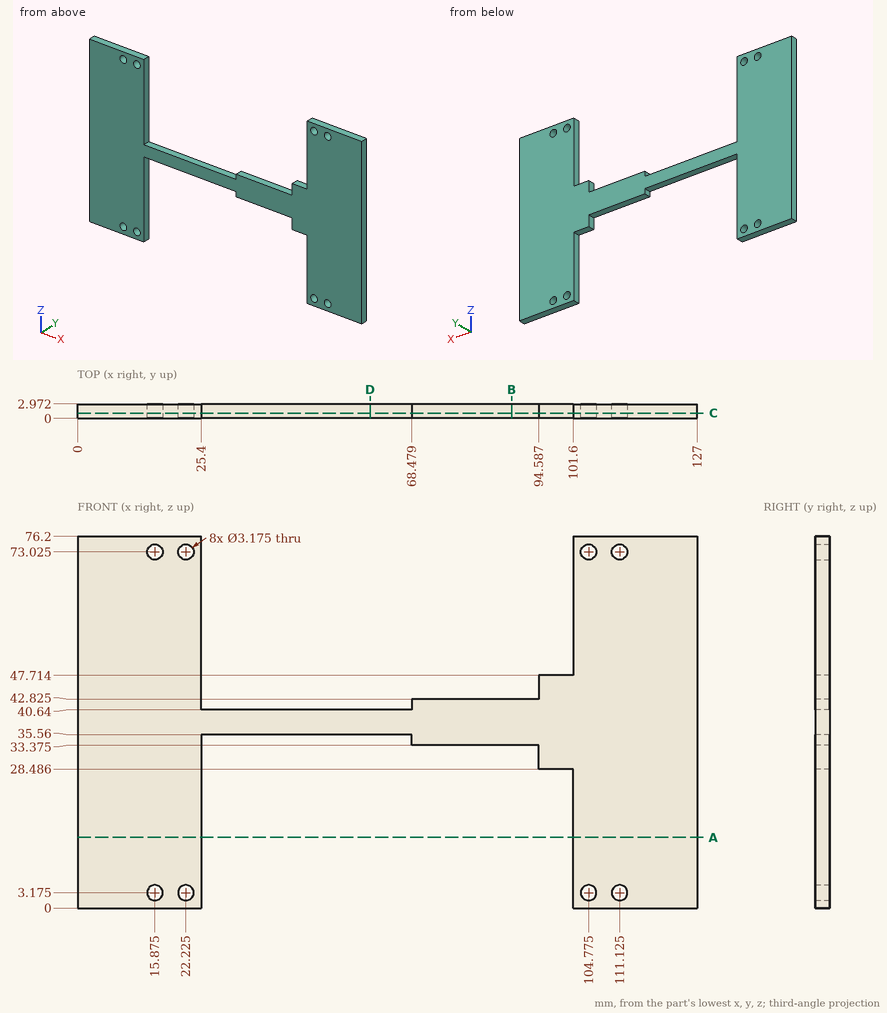
Study the drawing (mm; zero at the part's minimum x, y, z) and answer. Give positions to 0.01 mm unless a question says otherwise; leave off trailing zeros. Write each loop counter-clockwise with the first axis right and the second up, starting at its lowest first coordinate (ties: lowest second). Pieces come first, ordered by that corner, then holes.
Item 1: Flat-ended cylindrical pins translate along their axes: P1, Ø0.9, axis at x = 80, y = 2, coming from the +Z side (3 decimals); P2, Ø1.9, axis at x = 15.875, z = 73.025, coming from the +Y side. Find the tip coordinate at first contact, or state that the pin passes through.
Item 2: Section C-C, the plane y = 1.1 is taken. Count the separate pieces of the cut face and the enclosed holes in it, plus the area to 3 significant figures.
Item 3: Section A-A, the plane z = 14.5 is taken. Write down the section's boundary in (x, y), plus the area to 3 significant figures.
Item 4: Section D-D, the plane x = 60 is taken. Write down the section's boundary in (y, z).
Item 5: Find the intervals of material crossed by line 1 along X through (y, z) = (0.2, 15.5); line 2 along Z through (x, y) = (110, 1.3) (1 decimal); line 3 along X through (y, z) = (1.95, 3.5), in increasing order.
Item 6: Section B-B, the plane x = 89 is taken. Write down the section's boundary in (y, z) (1 decimal), plus the area to 3 significant figures.
Completed:
1. P1: stops at z = 42.825
1. P2: passes through
2. separate pieces: 1
2. enclosed holes: 8
2. area: 4,410 mm2
3. outline: (0, 0) - (25.4, 0) - (25.4, 2.97) - (0, 2.97) - close; (101.6, 0) - (127, 0) - (127, 2.97) - (101.6, 2.97) - close
3. area: 151 mm2
4. outline: (0, 35.56) - (2.97, 35.56) - (2.97, 40.64) - (0, 40.64) - close
5. line 1: x = 0 to 25.4, 101.6 to 127
5. line 2: z = 0 to 2.1, 4.3 to 71.9, 74.1 to 76.2
5. line 3: x = 0 to 14.32, 17.43 to 20.67, 23.78 to 25.4, 101.6 to 103.22, 106.33 to 109.57, 112.68 to 127
6. outline: (0, 33.4) - (3, 33.4) - (3, 42.8) - (0, 42.8) - close
6. area: 28.1 mm2
